Build history of the part. All positions in model axes, mm. A direction names the side the tool comes from. Give positions to 0.01 mm unless a question says otherwise; leave off trailing zeros. Order: outer loops, then holes, each group sorted by start corner. A loop starts at its lowest first (then second) coordinate and runs counter-clockwise, first axis right, second up. Notation, with made-up numbers: (18.25, -29.5) -> (59.25, -29.5) arc R17 cw to (59.25, -8.5) -> close; hole circle Ø2 at (-8.75, 51.25). An arc over 180 degrees is marked (long way). Write item = value, one per line. Start each with the question number.
from build123d import *

# Parameters (mm, degrees)
BOSS_EXTRUDE1_DEPTH = 29.5
CUT_EXTRUDE1_START  = -25
SKETCH2_R           = 22.247000374
CUT_EXTRUDE1_DEPTH  = 25
BOSS_EXTRUDE2_DEPTH = 2
CUT_EXTRUDE2_DEPTH  = 135.751896149
SKETCH5_R           = 1.775
CUT_EXTRUDE4_DEPTH  = 5.5
SKETCH6_R           = 1
CUT_EXTRUDE5_DEPTH  = 136.658849751


with BuildPart() as part:
    # Sketch1 → Boss-Extrude1 (new body)
    with BuildSketch(Plane(origin=(15, 0, 0), x_dir=(0, 0, -1), z_dir=(1, 0, 0))):
        with BuildLine():
            Line((11.711350424, 51.059854885), (11.569757763, 53.200462368))
            ThreePointArc((11.569757763, 53.200462368), (7.502659229, 61.435263917), (-1.19609774, 64.382274981))
            Line((-1.19609774, 64.382274981), (-13.169931797, 63.590253536))
            ThreePointArc((-13.169931797, 63.590253536), (-31.030401227, 77.615886129), (-53.600949688, 75.108879931))
            Line((-53.600949688, 75.108879931), (-83.257445184, 58.954243603))
            Line((-83.257445184, 58.954243603), (-95.231279241, 58.162222158))
            ThreePointArc((-95.231279241, 58.162222158), (-103.466080789, 54.095123625), (-106.413091853, 45.396366656))
            Line((-106.413091853, 45.396366656), (-106.271499192, 43.255759172))
            ThreePointArc((-106.271499192, 43.255759172), (-102.204400659, 35.020957624), (-93.50564369, 32.07394656))
            Line((-93.50564369, 32.07394656), (-81.531809632, 32.865968005))
            Line((-81.531809632, 32.865968005), (-50.005875623, 20.758305769))
            ThreePointArc((-50.005875623, 20.758305769), (-27.30176025, 21.246038307), (-11.444296246, 37.501977938))
            Line((-11.444296246, 37.501977938), (0.529537812, 38.293999383))
            ThreePointArc((0.529537812, 38.293999383), (8.76433936, 42.361097916), (11.711350424, 51.059854885))
        make_face()
        with BuildLine():
            Line((3.217758765, 50.677202056), (3.09976488, 52.461041626))
            ThreePointArc((3.09976488, 52.461041626), (-0.289483897, 59.323376249), (-7.538448038, 61.779218803))
            Line((-7.538448038, 61.779218803), (-17.516643086, 61.119200932))
            ThreePointArc((-17.516643086, 61.119200932), (-32.400367611, 72.807228093), (-51.209157995, 70.718056262))
            Line((-51.209157995, 70.718056262), (-75.922904242, 57.255859321))
            Line((-75.922904242, 57.255859321), (-85.901099289, 56.595841451))
            ThreePointArc((-85.901099289, 56.595841451), (-92.763433913, 53.206592673), (-95.219276466, 45.957628532))
            Line((-95.219276466, 45.957628532), (-95.101282582, 44.173788963))
            ThreePointArc((-95.101282582, 44.173788963), (-91.712033804, 37.311454339), (-84.463069663, 34.855611786))
            Line((-84.463069663, 34.855611786), (-74.484874616, 35.515629656))
            Line((-74.484874616, 35.515629656), (-48.213262941, 25.425911127))
            ThreePointArc((-48.213262941, 25.425911127), (-29.293166796, 25.832354908), (-16.07861346, 39.378971267))
            Line((-16.07861346, 39.378971267), (-6.100418412, 40.038989138))
            ThreePointArc((-6.100418412, 40.038989138), (0.761916211, 43.428237915), (3.217758765, 50.677202056))
        make_face(mode=Mode.SUBTRACT)
    extrude(amount=-BOSS_EXTRUDE1_DEPTH)

    # Sketch2 → Cut-Extrude1 (cut)
    with BuildSketch(Plane(origin=(15, 0, 0), x_dir=(0, 0, -1), z_dir=(1, 0, 0)).offset(CUT_EXTRUDE1_START)):
        with Locations((-38.176329446, 53.173227685)):
            Circle(SKETCH2_R)
        with Locations((-37.60491264, 44.534509548)):
            Circle(SKETCH2_R)
    extrude(amount=CUT_EXTRUDE1_DEPTH, mode=Mode.SUBTRACT)

    # Sketch3 → Boss-Extrude2 (add)
    with BuildSketch(Plane.ZY.offset(14.5)):
        with BuildLine():
            Line((83.257445184, 58.954243603), (53.600949688, 75.108879931))
            ThreePointArc((53.600949688, 75.108879931), (31.030401227, 77.615886129), (13.169931797, 63.590253536))
            Line((13.169931797, 63.590253536), (1.19609774, 64.382274981))
            ThreePointArc((1.19609774, 64.382274981), (-7.502659229, 61.435263917), (-11.569757763, 53.200462368))
            Line((-11.569757763, 53.200462368), (-11.711350424, 51.059854885))
            ThreePointArc((-11.711350424, 51.059854885), (-8.76433936, 42.361097916), (-0.529537812, 38.293999383))
            Line((-0.529537812, 38.293999383), (11.444296246, 37.501977938))
            ThreePointArc((11.444296246, 37.501977938), (27.30176025, 21.246038307), (50.005875623, 20.758305769))
            Line((50.005875623, 20.758305769), (81.531809632, 32.865968005))
            Line((81.531809632, 32.865968005), (93.50564369, 32.07394656))
            ThreePointArc((93.50564369, 32.07394656), (102.204400659, 35.020957624), (106.271499192, 43.255759172))
            Line((106.271499192, 43.255759172), (106.413091853, 45.396366656))
            ThreePointArc((106.413091853, 45.396366656), (103.466080789, 54.095123625), (95.231279241, 58.162222158))
            Line((95.231279241, 58.162222158), (83.257445184, 58.954243603))
        make_face()
        with BuildLine():
            ThreePointArc((74.264539557, 44.823732686), (72.076754007, 50.799817892), (66.100668801, 48.612032342))
            ThreePointArc((66.100668801, 48.612032342), (68.288454351, 42.635947136), (74.264539557, 44.823732686))
        make_face(mode=Mode.SUBTRACT)
    extrude(amount=BOSS_EXTRUDE2_DEPTH)

    # Sketch4 → Cut-Extrude2 (cut, through all)
    with BuildSketch(Plane(origin=(-10, 0, 0), x_dir=(0, 0, -1), z_dir=(1, 0, 0))):
        with BuildLine():
            ThreePointArc((-73.418847587, 51.830670487), (-72.378344752, 51.449752714), (-71.997426979, 52.490255549))
            ThreePointArc((-71.997426979, 52.490255549), (-73.037929814, 52.871173322), (-73.418847587, 51.830670487))
        make_face()
        with BuildLine():
            ThreePointArc((-64.029313371, 49.573208149), (-65.069816206, 49.954125922), (-65.450733979, 48.913623087))
            ThreePointArc((-65.450733979, 48.913623087), (-64.410231144, 48.532705314), (-64.029313371, 49.573208149))
        make_face()
        with BuildLine():
            ThreePointArc((-74.914474378, 44.522141941), (-75.954977214, 44.903059714), (-76.335894987, 43.862556879))
            ThreePointArc((-76.335894987, 43.862556879), (-75.295392151, 43.481639106), (-74.914474378, 44.522141941))
        make_face()
        with BuildLine():
            ThreePointArc((-66.946360771, 41.605094541), (-67.986863606, 41.986012314), (-68.367781379, 40.945509479))
            ThreePointArc((-68.367781379, 40.945509479), (-67.327278544, 40.564591706), (-66.946360771, 41.605094541))
        make_face()
    extrude(amount=-CUT_EXTRUDE2_DEPTH, mode=Mode.SUBTRACT)

    # Sketch5 → Cut-Extrude4 (cut)
    with BuildSketch(Plane(origin=(-10, 0, 0), x_dir=(0, 0, -1), z_dir=(1, 0, 0))):
        with Locations((-72.708137283, 52.160463018)):
            Circle(SKETCH5_R)
        with Locations((-64.740023675, 49.243415618)):
            Circle(SKETCH5_R)
        with Locations((-67.657071075, 41.27530201)):
            Circle(SKETCH5_R)
        with Locations((-75.625184683, 44.19234941)):
            Circle(SKETCH5_R)
    extrude(amount=-CUT_EXTRUDE4_DEPTH, mode=Mode.SUBTRACT)

    # Sketch6 → Cut-Extrude5 (cut, through all)
    with BuildSketch(Plane(origin=(-14.5, 0, 0), x_dir=(0, 0, -1), z_dir=(1, 0, 0))):
        with Locations(Location((-29.729663164, 34.080294384, 0), (0, 0, 90))):
            Circle(SKETCH6_R)
        with Locations(Location((-53.93384306, 39.243401547, 0), (0, 0, 90))):
            Circle(SKETCH6_R)
        with Locations(Location((-24.566556001, 58.28447428, 0), (0, 0, 90))):
            Circle(SKETCH6_R)
        with Locations(Location((-48.770735897, 63.447581443, 0), (0, 0, 90))):
            Circle(SKETCH6_R)
    extrude(amount=-CUT_EXTRUDE5_DEPTH, mode=Mode.SUBTRACT)


solid = part.part
(1) Flat gauge pins, fed straight in: P1, Ø3, axis at y = 44.19, z = 75.63, coming from the +X side; P2, Ø5, axis at x = 3, z = 22, coming from the -Y side; P3, Ø2.5, axis at y = 63.45, z = 48.77, coming from the +X side. Where does each tip first touch, or does it go through?
(2) Wall check: line 1 (X direction, y = 50.5, z = 42); line 2 (Y direction, x = 12.5, z = 21); line 3 (Y direction, x = 14, z = 4). Give the ranges that are in metal, low to high. Write a range as [from, to].
(3) Cut at A-A, the plane x = -13. Give the cut face in (y, z), plus the area to 3 significant figures.
(4) 3-axis set-ups, long thin cutter, end or side, ignore diameter. For faces 1 (the face through (-0.53, 32.476, 87.435)), 2 (the face through (-14.5, 49, 45)): which of +Z, -Z, +X, -X, +Y, -Y reach the whole face in a straight line?
(5) Mould opens along Z. For faces 3 (the face through (0.457, 59.25, 0.207)), 4 (the face through (-0.53, 52.15, -11.64)) say: released by +Z, released by -Z, zero draft, split by the parting line, or undercut.
(6) Cut at B-B, the plane y = 30. Give the cut face in (x, z).
(7) Cut at C-C, the plane x = 1. Give the cut face in (y, z), plus the area to 3 significant figures.
Results:
q1.P1 = -15.5
q1.P2 = 22.64
q1.P3 = -14.5
q2.line_1 = [-16.5, -14.5]
q2.line_2 = [24.95, 29.73], [67.31, 72.57]
q2.line_3 = [37.99, 40.41], [61.38, 64.2]
q3.outline = (20.76, 50.01) arc R30 ccw to (37.5, 11.44) -> (38.29, -0.53) arc R12 ccw to (51.06, -11.71) -> (53.2, -11.57) arc R12 ccw to (64.38, 1.2) -> (63.59, 13.17) arc R30 ccw to (75.11, 53.6) -> (58.95, 83.26) -> (58.16, 95.23) arc R12 ccw to (45.4, 106.41) -> (43.26, 106.27) arc R12 ccw to (32.07, 93.51) -> (32.87, 81.53) -> close; hole (25.43, 48.21) arc R25 ccw to (39.38, 16.08) -> (40.04, 6.1) arc R10 ccw to (50.68, -3.22) -> (52.46, -3.1) arc R10 ccw to (61.78, 7.54) -> (61.12, 17.52) arc R25 ccw to (70.72, 51.21) -> (57.26, 75.92) -> (56.6, 85.9) arc R10 ccw to (45.96, 95.22) -> (44.17, 95.1) arc R10 ccw to (34.86, 84.46) -> (35.52, 74.48) -> close
q3.area = 1,360 mm2
q4.face_1 = +X, -X, -Y
q4.face_2 = +X
q5.face_3 = undercut
q5.face_4 = released by -Z
q6.outline = (-16.5, 15.84) -> (15, 15.84) -> (15, 20.76) -> (-10, 20.76) -> (-10, 22.73) -> (-14.5, 22.73) -> (-14.5, 60.12) -> (15, 60.12) -> (15, 74.07) -> (-16.5, 74.07) -> close
q7.outline = (20.76, 50.01) arc R30 ccw to (37.5, 11.44) -> (38.29, -0.53) arc R12 ccw to (51.06, -11.71) -> (53.2, -11.57) arc R12 ccw to (64.38, 1.2) -> (63.59, 13.17) arc R30 ccw to (75.11, 53.6) -> (58.95, 83.26) -> (58.16, 95.23) arc R12 ccw to (45.4, 106.41) -> (43.26, 106.27) arc R12 ccw to (32.07, 93.51) -> (32.87, 81.53) -> close; hole (26.18, 50.18) arc R22.25 ccw to (39.39, 15.96) -> (40.04, 6.1) arc R10 ccw to (50.68, -3.22) -> (52.46, -3.1) arc R10 ccw to (61.78, 7.54) -> (61.13, 17.4) arc R22.25 ccw to (69.71, 53.06) -> (57.26, 75.92) -> (56.6, 85.9) arc R10 ccw to (45.96, 95.22) -> (44.17, 95.1) arc R10 ccw to (34.86, 84.46) -> (35.52, 74.48) -> close
q7.area = 1,260 mm2
